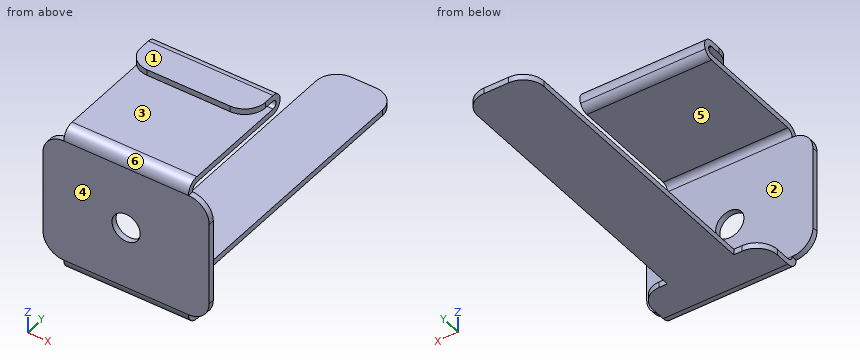
```python
from build123d import *

# Parameters (mm, degrees)
SKETCH1_W             = 20
SKETCH1_H             = 15
BASE_FLANGE1_DEPTH    = 0.7
EDGE_FLANGE1_DEPTH    = 15
SKETCH7_W             = 8
SKETCH7_H             = 35
TAB1_DEPTH            = 0.7
EDGE_FLANGE2_DEPTH    = 15
HEM1_START            = -7.5
HEM1_DEPTH            = 15
HEM1_2_DEPTH          = 15
SKETCH13_R            = 1.7
CUT_EXTRUDE1_DEPTH    = 0.7
BREAK_CORNER2_START   = -8.9366
BREAK_CORNER2_DEPTH   = 0.7
BREAK_CORNER2_START_2 = 9.9366
BREAK_CORNER2_2_DEPTH = 0.7
BREAK_CORNER2_START_3 = -0.7
BREAK_CORNER2_3_DEPTH = 0.7


# Read off the part's stored shape, not the designer's step: Hem1, Break-Corner2
# Sheet-metal steps are written as plain solids
with BuildPart() as part:
    # Sketch1 → Base-Flange1 (new body)
    with BuildSketch(Plane(origin=(0, 0, 0), x_dir=(1, 0, 0), z_dir=(0, 1, 0))):
        Rectangle(SKETCH1_W, SKETCH1_H)
    extrude(amount=-BASE_FLANGE1_DEPTH)

    # Edge-Flange1 section (across the edge) → Edge-Flange1 (add)
    with BuildSketch(Plane(origin=(7.5, 0, -8.2366), x_dir=(0, 0, 1), z_dir=(-1, 0, 0))):
        with BuildLine():
            Line((-0.7, 0.7366), (-0.7, 5))
            Line((-0.7, 5), (0, 5))
            Line((0, 5), (0, 0.7366))
            ThreePointArc((0, 0.7366), (0.215745145, 0.215745145), (0.7366, 0))
            Line((0.7366, 0), (0.7366, -0.7))
            ThreePointArc((0.7366, -0.7), (-0.279229602, -0.279229602), (-0.7, 0.7366))
        make_face()
    extrude(amount=EDGE_FLANGE1_DEPTH)

    # Sketch7 → Tab1 (add)
    with BuildSketch(Plane.XY.offset(-8.2366)):
        with Locations((0, 22.5)):
            Rectangle(SKETCH7_W, SKETCH7_H)
    extrude(amount=-TAB1_DEPTH)

    # Edge-Flange2 section (across the edge) → Edge-Flange2 (add)
    with BuildSketch(Plane(origin=(-7.5, 0, 8.2366), x_dir=(0, 0, -1), z_dir=(1, 0, 0))):
        with BuildLine():
            Line((-0.7, 0.7366), (-0.7, 15))
            Line((-0.7, 15), (0, 15))
            Line((0, 15), (0, 0.7366))
            ThreePointArc((0, 0.7366), (0.215745145, 0.215745145), (0.7366, 0))
            Line((0.7366, 0), (0.7366, -0.7))
            ThreePointArc((0.7366, -0.7), (-0.279229602, -0.279229602), (-0.7, 0.7366))
        make_face()
    extrude(amount=EDGE_FLANGE2_DEPTH)

    # Hem1 outline → Hem1 (cut)
    with BuildSketch(Plane.YZ.offset(HEM1_START)):
        with BuildLine():
            Line((15, 8.9366), (14.890871211, 8.9366))
            ThreePointArc((14.890871211, 8.9366), (14.44807407, 8.426649506), (13.8, 8.2366))
            Line((13.8, 8.2366), (15, 8.2366))
            Line((15, 8.2366), (15, 8.9366))
        make_face()
    extrude(amount=HEM1_DEPTH, mode=Mode.SUBTRACT)

    # Hem1 2 outline → Hem1 2 (add)
    with BuildSketch(Plane.YZ.offset(HEM1_START)):
        with BuildLine():
            Line((10, 10.6366), (10, 9.9366))
            Line((10, 9.9366), (13.8, 9.9366))
            ThreePointArc((13.8, 9.9366), (14.3, 9.4366), (13.8, 8.9366))
            Line((13.8, 8.9366), (14.890871211, 8.9366))
            ThreePointArc((14.890871211, 8.9366), (14.809950494, 10.08467407), (13.8, 10.6366))
            Line((13.8, 10.6366), (10, 10.6366))
        make_face()
    extrude(amount=HEM1_2_DEPTH)

    # Sketch13 → Cut-Extrude1 (cut)
    with BuildSketch(Plane(origin=(0, 0, 0), x_dir=(1, 0, 0), z_dir=(0, 1, 0))):
        with Locations(Location((0, 0, 0), (0, 0, 270))):
            Circle(SKETCH13_R)
    extrude(amount=-CUT_EXTRUDE1_DEPTH, mode=Mode.SUBTRACT)

    # Break-Corner2 outline → Break-Corner2 (cut)
    with BuildSketch(Plane.XY.offset(BREAK_CORNER2_START)):
        with BuildLine():
            Line((7.5, 5), (5.001, 5))
            ThreePointArc((5.001, 5), (6.768059846, 4.268059846), (7.5, 2.501))
            Line((7.5, 2.501), (7.5, 5))
        make_face()
        with BuildLine():
            ThreePointArc((-7.5, 2.501), (-6.768059846, 4.268059846), (-5.001, 5))
            Line((-5.001, 5), (-7.5, 5))
            Line((-7.5, 5), (-7.5, 2.501))
        make_face()
        with BuildLine():
            Line((-4, 40), (-4, 37.501))
            ThreePointArc((-4, 37.501), (-3.268059846, 39.268059846), (-1.501, 40))
            Line((-1.501, 40), (-4, 40))
        make_face()
        with BuildLine():
            ThreePointArc((1.501, 40), (3.268059846, 39.268059846), (4, 37.501))
            Line((4, 37.501), (4, 40))
            Line((4, 40), (1.501, 40))
        make_face()
    extrude(amount=BREAK_CORNER2_DEPTH, mode=Mode.SUBTRACT)

    # Break-Corner2 2 outline → Break-Corner2 2 (cut)
    with BuildSketch(Plane.XY.offset(BREAK_CORNER2_START_2)):
        with BuildLine():
            ThreePointArc((7.5, 12.499), (6.768059846, 10.731940154), (5.001, 10))
            Line((5.001, 10), (7.5, 10))
            Line((7.5, 10), (7.5, 12.499))
        make_face()
        with BuildLine():
            ThreePointArc((-5.001, 10), (-6.768059846, 10.731940154), (-7.5, 12.499))
            Line((-7.5, 12.499), (-7.5, 10))
            Line((-7.5, 10), (-5.001, 10))
        make_face()
    extrude(amount=BREAK_CORNER2_2_DEPTH, mode=Mode.SUBTRACT)

    # Break-Corner2 3 outline → Break-Corner2 3 (cut)
    with BuildSketch(Plane(origin=(0, 0, 0), x_dir=(1, 0, 0), z_dir=(0, 1, 0)).offset(BREAK_CORNER2_START_3)):
        with BuildLine():
            ThreePointArc((7.501, 7.5), (9.268059846, 6.768059846), (10, 5.001))
            Line((10, 5.001), (10, 7.5))
            Line((10, 7.5), (7.501, 7.5))
        make_face()
        with BuildLine():
            ThreePointArc((10, -5.001), (9.268059846, -6.768059846), (7.501, -7.5))
            Line((7.501, -7.5), (10, -7.5))
            Line((10, -7.5), (10, -5.001))
        make_face()
        with BuildLine():
            Line((-10, 7.5), (-10, 5.001))
            ThreePointArc((-10, 5.001), (-9.268059846, 6.768059846), (-7.501, 7.5))
            Line((-7.501, 7.5), (-10, 7.5))
        make_face()
        with BuildLine():
            ThreePointArc((-7.501, -7.5), (-9.268059846, -6.768059846), (-10, -5.001))
            Line((-10, -5.001), (-10, -7.5))
            Line((-10, -7.5), (-7.501, -7.5))
        make_face()
    extrude(amount=BREAK_CORNER2_3_DEPTH, mode=Mode.SUBTRACT)


solid = part.part
```
Model file for the job. Use its own axes, mm. Face numbers are marked on the shaded views. A direction names the side the tool comes from. Give positions to 0.01 mm unless a question says otherwise; leave off trailing zeros. Loops run counter-clockwise (first coordinate to the right, second up) from the corner with the lowest first, then second, coordinate; pieces in that order, holes last. Notation, with made-up numbers: M 56.5,66 L 92.5,66 A26 ccw 92.5,87 Z; hole C 35.5,-3 d4. An arc over 180 degrees is marked long. Use one line per item in the form item = value.
Item 1: Drill centre lines: L1, parallel to X at y = -0.35, z = 0; L2, parallel to Z at x = 2, y = 8.5; L3, parallel to Y at x = -3.75, z = 6.5. Where is each one in solid material? Low to high.
Filled in:
L1 = -10 to -1.7, 1.7 to 10
L2 = -8.94 to -8.24, 8.24 to 8.94
L3 = -0.7 to 0
Item 2: Two-plate mould, pull along Z, no slides. Class the marked faces 3, 4, 5 and 6: released by +Z, released by -Z, zero draft, split by the parting line, or undercut.
Filled in:
face_3 = undercut
face_4 = zero draft
face_5 = undercut
face_6 = released by +Z
Item 3: Which spindle directions (+Z, -Z, +X, -X, +Y, -Y) get a long thin tool onto all of the face, cutting with end or side? Do the marked faces 1 and 2. Say none if no direction does.
Filled in:
face_1 = +Z, +X, -X, +Y, -Y
face_2 = +X, -X, +Y
Item 4: Slice it at A-A on z = 0. List the corners of the cut face in (x, y), and give its area (3 significant figures).
Filled in:
outline = M -10,-0.7 L -1.7,-0.7 L -1.7,0 L -10,0 Z; M 1.7,-0.7 L 10,-0.7 L 10,0 L 1.7,0 Z
area = 11.6 mm^2
Item 5: Slice it at C-C on x = -2.25. List the corners of the cut face in (y, z).
Filled in:
outline = M -0.7,-7.5 A1.44 ccw 0.74,-8.94 L 39.89,-8.94 L 39.89,-8.24 L 0.74,-8.24 A0.74 cw 0,-7.5 L 0,7.5 A0.74 cw 0.74,8.24 L 13.8,8.24 A1.2 ccw 13.8,10.64 L 10,10.64 L 10,9.94 L 13.8,9.94 A0.5 cw 13.8,8.94 L 0.74,8.94 A1.44 ccw -0.7,7.5 Z
Item 6: Slice it at B-B on x = 0. List the corners of the cut face in (y, z), and give its area (3 significant figures).
Filled in:
outline = M -0.7,-7.5 A1.44 ccw 0.74,-8.94 L 40,-8.94 L 40,-8.24 L 0.74,-8.24 A0.74 cw 0,-7.5 L 0,-1.7 L -0.7,-1.7 Z; M -0.7,1.7 L 0,1.7 L 0,7.5 A0.74 cw 0.74,8.24 L 13.8,8.24 A1.2 ccw 13.8,10.64 L 10,10.64 L 10,9.94 L 13.8,9.94 A0.5 cw 13.8,8.94 L 0.74,8.94 A1.44 ccw -0.7,7.5 Z
area = 51.7 mm^2
Item 7: Flat gauge pins, fed straight in: pin 1 Ø7.5 at (x, z) = (0, -0.5) entering from +Y; pin 2 Ø1.6 at (y, z) = (1, -8.5) entering from -X; pin 3 Ø1.6 at (y, z) = (1.5, -8.5) entering from +X. Where does each tip first touch, or does it go through?
Filled in:
pin_1 = 0
pin_2 = -7.5
pin_3 = 7.5
Item 8: Slice it at D-D on y = 36. List the corners of the cut face in (x, z), and give its area (3 significant figures).
Filled in:
outline = M -4,-8.94 L 4,-8.94 L 4,-8.24 L -4,-8.24 Z
area = 5.60 mm^2
